Work out the finished part from the listing and answer in its coordinate system (mm). A direction names the side the tool comes from. Coordinates: 2 decimals unless noted, no trailing zeros. Order: outer loops, then holes, each group sorted by start corner. A loop starts at its lowest first (then second) coordinate and runs counter-clockwise, first axis right, second up. Notation, with made-up numbers: (69.25, 62.25) - (101.25, 62.25) arc R21 cw to (101.25, 84.25) - close; hole circle Ø3 at (-27, -16). An arc over 180 degrees is marked (long way). Answer as a JSON object with one key per item and string values. Group by question number.
1) A tool of negligible diameter and unlimited length cuts with its end or side. For faces 1 (the face through (0, 11, 42)), 2 (the face through (14, 0, 18.25)), 3 (the face through (8, 1, 48)), 4 (the face through (14.2, 2.5, 16.5)), from which of +Z, -Z, +X, -X, +Y, -Y can it reach the whole face along a straight path? Write none if from no direction.
2) Section C-C (z = 32) is taken. Give the vertices of the cut face in (x, y), plus the area to 3 significant figures.
3) Section B-B (z = -2.25) is taken. Give the vertices of the cut face in (x, y).
4) Section A-A (y = 0) is taken. Give the vertices of the cut face in (x, z), plus the area to 3 significant figures.
5) Each of these flat-tipped pins is pushed along its axis until it touches: P1, Ø10, axis at y = -0.5, z = 58, coming from the -X side; P2, Ø1.8, axis at x = -12, y = 0, coming from the +Z side; P3, Ø9, axis at y = 2.5, z = 40, coming from the +X side; P4, Ø1.3, axis at y = 0.5, z = -2, coming from the +X side. Where does it stop, or does it pass through?
6) Find the intervals of material crossed by line 1 along Y through (x, z) = (3.5, 32); line 2 along Z through (x, y) = (-0.1, 0); line 3 along Z through (x, y) = (-4, 3), in increasing order.
7) Section D-D (y = 4.5) is taken. Give the vertices of the cut face in (x, z).
Autodesk Inventor part; units mm, degrees
ref_plane "YZ Plane" through (0, 0, 0) normal (1, 0, 0) x (0, 1, 0)
ref_plane "XZ Plane" through (0, 0, 0) normal (0, 1, 0) x (-1, 0, 0)
ref_plane "XY Plane" through (0, 0, 0) normal (0, 0, 1) x (1, 0, 0)
sketch "Эскиз1" plane through (0, 0, 0) normal (0, 0, 1) x (1, 0, 0)
  line L0 (9.5, -11) -> (-9.5, -11)
  line L1 (-9.5, -11) -> (-9.5, 11)
  line L2 (-9.5, 11) -> (9.5, 11)
  line L3 (9.5, 11) -> (9.5, -11)
  line L4 (9.5, -11) -> (-9.5, 11) construction
  line L5 (-9.5, -11) -> (9.5, 11) construction
  point P0 (0, 0)
  dimension "d0" = 19
  dimension "d1" = 22
extrude "Выдавливание1" add sketch "Эскиз1" along normal blind 37
sketch "Эскиз2" plane through (0, 0, 37) normal (0, 0, 1) x (1, 0, 0)
  circle A0 centre (0, 0) radius 11
  line L0 (8.5, -20.0649) -> (-8.5, -20.0649)
  line L1 (-8.5, -20.0649) -> (-8.5, 20.0649)
  line L2 (-8.5, 20.0649) -> (8.5, 20.0649)
  line L3 (8.5, 20.0649) -> (8.5, -20.0649)
  line L4 (8.5, -20.0649) -> (-8.5, 20.0649) construction
  line L5 (-8.5, -20.0649) -> (8.5, 20.0649) construction
  point P0 (8.5, -6.9821)
  point P1 (8.5, 6.9821)
  point P2 (-8.5, 6.9821)
  point P3 (-8.5, -6.9821)
  dimension "d4" = 22
  dimension "d5" = 17
extrude "Выдавливание2" add sketch "Эскиз2" along normal blind 11 contours L3 A0 L1
sketch "Эскиз3" plane through (9.5, -11, 0) normal (1, 0, 0) x (0, 0, -1)
  circle A0 centre (-32, 19.5) radius 1.5
  line L0 (-37, 0) -> (-37, 22)
  line L1 (0, 22) -> (-37, 22)
  line L2 (-37, 4.0179) -> (-37, 17.9821)
  line L3 (-37, 11) -> (0, 11)
  line L4 (0, 0) -> (0, 22)
  circle A1 centre (-32, 2.5) radius 1.5
  dimension "d8" = 3
  dimension "d9" = 5
  dimension "d10" = 2.5
extrude "Выдавливание3" cut sketch "Эскиз3" against normal through all contours A0 | A1
sketch "Эскиз4" plane through (9.5, -11, 0) normal (1, 0, 0) x (0, 0, -1)
  circle A0 centre (-16.5, 11) radius 2.5
  line L0 (0, 0) -> (0, 22)
  line L1 (0, 0) -> (-37, 0)
  line L2 (-14.75, 6.8216) -> (-18.25, 6.8216)
  line L3 (-18.25, 6.8216) -> (-18.25, 15.1784)
  line L4 (-18.25, 15.1784) -> (-14.75, 15.1784)
  line L5 (-14.75, 15.1784) -> (-14.75, 6.8216)
  line L6 (-14.75, 6.8216) -> (-18.25, 15.1784) construction
  line L7 (-18.25, 6.8216) -> (-14.75, 15.1784) construction
  point P0 (0, 11)
  point P1 (-14.75, 9.2146)
  point P2 (-14.75, 12.7854)
  point P3 (-18.25, 12.7854)
  point P4 (-18.25, 9.2146)
  dimension "d13" = 5
  dimension "d14" = 16.5
  dimension "d15" = 11
  dimension "d16" = 3.5
extrude "Выдавливание4" add sketch "Эскиз4" along normal blind 9.5 and the other way blind 28.5 contours L5 A0 L3
sketch "Эскиз5" plane through (0, 0, 48) normal (0, 0, 1) x (1, 0, 0)
  circle A0 centre (0, 0) radius 9.75
  line L0 (7.5, 17.2473) -> (-7.5, 17.2473)
  line L1 (-7.5, 17.2473) -> (-7.5, -17.2473)
  line L2 (-7.5, -17.2473) -> (7.5, -17.2473)
  line L3 (7.5, -17.2473) -> (7.5, 17.2473)
  line L4 (7.5, 17.2473) -> (-7.5, -17.2473) construction
  line L5 (-7.5, 17.2473) -> (7.5, -17.2473) construction
  point P0 (7.5, -6.23)
  point P1 (7.5, 6.23)
  point P2 (-7.5, 6.23)
  point P3 (-7.5, -6.23)
  dimension "d21" = 19.5
  dimension "d22" = 15
extrude "Выдавливание5" add sketch "Эскиз5" along normal blind 17 contours L3 A0 L1
fillet "Сопряжение1" radius 3.5 2 edges at (0, -11, 0) (0, 11, 0)
sketch "Эскиз6" plane through (0, 0, 0) normal (0, 0, -1) x (-1, 0, 0)
  line L0 (-1.25, 2.5) -> (1.25, 2.5)
  line L1 (1.25, 2.5) -> (1.25, -2.5)
  line L2 (1.25, -2.5) -> (-1.25, -2.5)
  line L3 (-1.25, -2.5) -> (-1.25, 2.5)
  line L4 (-1.25, 2.5) -> (1.25, -2.5) construction
  line L5 (1.25, 2.5) -> (-1.25, -2.5) construction
  point P0 (0, 0)
  dimension "d26" = 2.5
  dimension "d27" = 5
extrude "Выдавливание6" add sketch "Эскиз6" along normal blind 4.5
sketch "Эскиз7" plane through (-1.25, -2.5, 0) normal (-1, 0, 0) x (0, 0, 1)
  line L0 (0, 0) -> (-4.5, 0)
  line L1 (0, 5) -> (-4.5, 5)
  line L2 (-4.5, 0) -> (-4.5, 5)
  line L3 (-4.5, 2.5) -> (0, 2.5)
  circle A0 centre (-2.25, 2.5) radius 1.5
  dimension "d31" = 3
extrude "Выдавливание7" cut sketch "Эскиз7" against normal through all
properties part number "мотор лол"
Report:
{
 "1": {"face 1": "+Z, +Y", "face 2": "+Z, +X, +Y, -Y", "face 3": "+Z", "face 4": "+X, +Y"},
 "2": {"outline": "(-9.5, -11) - (9.5, -11) - (9.5, -10) - (-9.5, -10) - close; (-9.5, -7) - (9.5, -7) - (9.5, 7) - (-9.5, 7) - close; (-9.5, 10) - (9.5, 10) - (9.5, 11) - (-9.5, 11) - close", "area": "304 mm²"},
 "3": {"outline": "(-1.25, -2.5) - (1.25, -2.5) - (1.25, -1.5) - (-1.25, -1.5) - close; (-1.25, 1.5) - (1.25, 1.5) - (1.25, 2.5) - (-1.25, 2.5) - close"},
 "4": {"outline": "(-19, 14.75) - (-9.5, 14.75) - (-9.5, 0) - (-1.25, 0) - (-1.25, -0.75) - (1.25, -0.75) - (1.25, 0) - (9.5, 0) - (9.5, 14.75) - (19, 14.75) - (19, 18.25) - (9.5, 18.25) - (9.5, 37) - (8.5, 37) - (8.5, 48) - (7.5, 48) - (7.5, 65) - (-7.5, 65) - (-7.5, 48) - (-8.5, 48) - (-8.5, 37) - (-9.5, 37) - (-9.5, 18.25) - (-19, 18.25) - close; (-1.25, -4.5) - (1.25, -4.5) - (1.25, -3.75) - (-1.25, -3.75) - close", "area": "1,220 mm²"},
 "5": {"P1": "stops at x = -7.5", "P2": "stops at z = 18.25", "P3": "stops at x = 9.5", "P4": "passes through"},
 "6": {"line 1": "y = -11 to -10, -7 to 7, 10 to 11", "line 2": "z = -4.5 to -3.75, -0.75 to 65", "line 3": "z = 0 to 65"},
 "7": {"outline": "(-9.5, 0) - (9.5, 0) - (9.5, 37) - (8.5, 37) - (8.5, 48) - (7.5, 48) - (7.5, 65) - (-7.5, 65) - (-7.5, 48) - (-8.5, 48) - (-8.5, 37) - (-9.5, 37) - close"}
}
